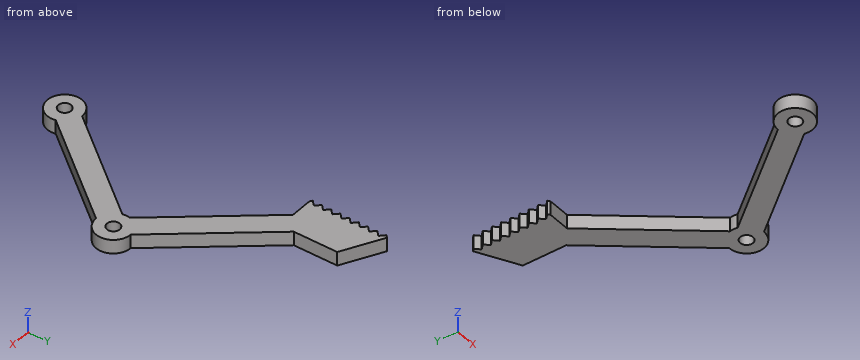
from build123d import *

# Parameters (mm, degrees)
BOSS_EXTRUDE1_DEPTH = 3.18
SKETCH2_R           = 1.47
CUT_EXTRUDE1_DEPTH  = 76.406636354


with BuildPart() as part:
    # Sketch1 → Boss-Extrude1 (new body)
    with BuildSketch(Plane.XY):
        with BuildLine():
            Line((0, 4), (18.75, 27.418742494))
            ThreePointArc((18.75, 27.418742494), (18.653123749, 28.293742494), (18.75, 29.168742494))
            Line((18.75, 29.168742494), (0, 52.587484988))
            Line((0, 52.587484988), (-5, 52.587484988))
            Line((-5, 52.587484988), (-5.530330085, 52.96527181))
            Line((-5.530330085, 52.96527181), (-4.469669914, 54.025931982))
            Line((-4.469669914, 54.025931982), (-5.530330085, 55.086592153))
            Line((-5.530330085, 55.086592153), (-4.469669914, 56.147252325))
            Line((-4.469669914, 56.147252325), (-5.530330086, 57.207912497))
            Line((-5.530330086, 57.207912497), (-4.469669914, 58.268572669))
            Line((-4.469669914, 58.268572669), (-5.530330086, 59.32923284))
            Line((-5.530330086, 59.32923284), (-4.469669914, 60.389893012))
            Line((-4.469669914, 60.389893012), (-5.530330086, 61.450553184))
            Line((-5.530330086, 61.450553184), (-4.469669914, 62.511213356))
            Line((-4.469669914, 62.511213356), (-5.530330086, 63.571873527))
            Line((-5.530330086, 63.571873527), (-4.469669914, 64.632533699))
            Line((-4.469669914, 64.632533699), (-5.530330086, 65.693193871))
            Line((-5.530330086, 65.693193871), (-4.469669914, 66.753854043))
            Line((-4.469669914, 66.753854043), (-5.530330086, 67.814514215))
            Line((-5.530330086, 67.814514215), (-4.469669914, 68.875174386))
            Line((-4.469669914, 68.875174386), (-5.530330086, 69.935834558))
            Line((-5.530330086, 69.935834558), (-5.000000002, 70.467435037))
            Line((-5.000000002, 70.467435037), (3.903123749, 65.712484988))
            Line((3.903123749, 65.712484988), (3.903123749, 55.712484988))
            Line((3.903123749, 55.712484988), (22.653123749, 32.293742494))
            ThreePointArc((22.653123749, 32.293742494), (26.653123749, 28.293742494), (22.653123749, 24.293742494))
            Line((22.653123749, 24.293742494), (3.903123749, 0.875))
            ThreePointArc((3.903123749, 0.875), (-2.5, -3.122498999), (0, 4))
        make_face()
    extrude(amount=BOSS_EXTRUDE1_DEPTH)

    # Sketch2 → Cut-Extrude1 (cut, through all)
    with BuildSketch(Plane.XY.offset(3.18)):
        with Locations((22.653123749, 28.293742494)):
            Circle(SKETCH2_R)
        Circle(SKETCH2_R)
    extrude(amount=-CUT_EXTRUDE1_DEPTH, mode=Mode.SUBTRACT)


solid = part.part
The listing builds one solid part. Answer for the finished solid, in the listing's coordinates (mm). Give positions to 0.01 mm unless a question says otherwise; leave off trailing zeros. Write each loop counter-clockwise with the first axis right and the second up, starting at its lowest first coordinate (ties: lowest second). Pieces come first, ordered by that corner, then holes.
Item 1: Section C-C, the plane x = 9 is taken. Write down the section's boundary in (y, z), plus the area to 3 significant figures.
Item 2: Section B-B, the plane z = 1.9 is taken. Count the separate pieces of the cut face and the enclosed holes in it, plus the area to 3 significant figures.
Item 3: Section D-D, the plane y = 41 is taken. Write down the section's boundary in (x, z).
Item 4: Find the intervals of material crossed by line 1 along Y through (x, z) = (1, 2.2); line 2 along Y through (x, z) = (17.5, 0.65); line 3 along Y through (x, z) = (18, 0.3), in increasing order.
Item 5: Section A-A, the plane y = 0 is taken. Write down the section's boundary in (x, z), plus the area to 3 significant figures.
Item 6: Flat-ended cylindrical pins translate along their axes: P1, Ø4.5, axis at x = 0, y = 0, coming from the -Z side; P2, Ø1.5, axis at y = 34, z = 1, coming from the +X side; P3, Ø1, axis at x = 4, z = 0.5, coming from the -Y side. Find the tip coordinate at first contact, or state that the pin passes through.
Completed:
1. outline: (7.24, 0) - (15.24, 0) - (15.24, 3.18) - (7.24, 3.18) - close; (41.35, 0) - (49.35, 0) - (49.35, 3.18) - (41.35, 3.18) - close
1. area: 50.9 mm2
2. separate pieces: 1
2. enclosed holes: 2
2. area: 510 mm2
3. outline: (9.28, 0) - (15.68, 0) - (15.68, 3.18) - (9.28, 3.18) - close
4. line 1: y = -3.87 to -1.08, 1.08 to 5.25, 51.34 to 67.26
4. line 2: y = 17.86 to 25.86, 30.73 to 38.73
4. line 3: y = 18.48 to 26.48, 30.11 to 38.11
5. outline: (-4, 0) - (-1.47, 0) - (-1.47, 3.18) - (-4, 3.18) - close; (1.47, 0) - (4, 0) - (4, 3.18) - (1.47, 3.18) - close
5. area: 16.1 mm2
6. P1: stops at z = 0
6. P2: stops at x = 21.89
6. P3: stops at y = -1.94
